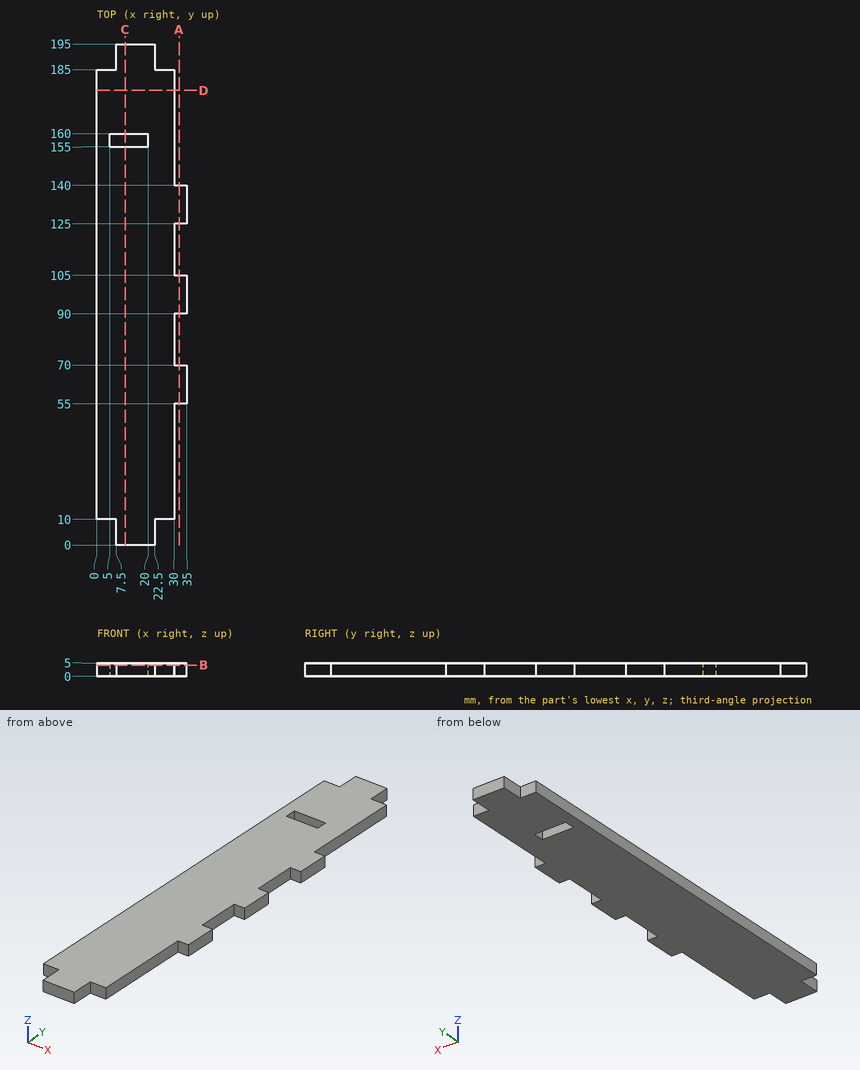
The figure shows three views and two pictorial views of one solid part (mm, origin at its lowest corner). Answer the questions. Give positions to 0.01 mm unless a question says otherwise; leave off trailing zeros. Loops run counter-clockwise (first coordinate to the right, second up) from the corner with the lowest first, then second, coordinate; pieces in that order, holes last. Notation, with made-up numbers: (-3, -3) -> (54, -3) arc R21 ccw to (54, 31) -> close; hole circle Ø9 at (73.25, 68). An arc over 180 degrees is marked (long way). Put each result on its own line as item: value. Start each with the question number.
Item 1: The part is cut by section C-C (x = 11). Give the vertices of the cut face in (y, z), then the cut area to 3 significant figures.
Item 2: The part is cut by section D-D (y = 177). Give the vertices of the cut face in (x, z), then the cut area to 3 significant figures.
Item 3: The part is cut by section B-B (z = 4.25). Give the vertices of the cut face in (x, y), then the cut area to 3 significant figures.
Item 4: Find the intervals of material crossed by L1, parallel to Y at x = 33.5, z = 4.3; L2, parallel to Y at x = 13.5, z = 1.8; L3, parallel to Y at x = 6, z = 1.6, in increasing order. Write a range as [from, to].
Item 5: Each of these flat-tipped pins is pushed along its axis until it touches: P1, Ø2.5, axis at x = 32, z = 3, coming from the -Y side; P2, Ø2, axis at y = 121, z = 4, coming from the +X side; P3, Ø1.5, axis at x = 28, z = 3, coming from the +Y side. Where does it stop, or does it pass through?
Item 6: The part is cut by section A-A (x = 32). Give the vertices of the cut face in (y, z).
Answers below:
1. outline: (0, 0) -> (155, 0) -> (155, 5) -> (0, 5) -> close; (160, 0) -> (195, 0) -> (195, 5) -> (160, 5) -> close
1. area: 950 mm2
2. outline: (0, 0) -> (30, 0) -> (30, 5) -> (0, 5) -> close
2. area: 150 mm2
3. outline: (0, 10) -> (7.5, 10) -> (7.5, 0) -> (22.5, 0) -> (22.5, 10) -> (30, 10) -> (30, 55) -> (35, 55) -> (35, 70) -> (30, 70) -> (30, 90) -> (35, 90) -> (35, 105) -> (30, 105) -> (30, 125) -> (35, 125) -> (35, 140) -> (30, 140) -> (30, 185) -> (22.5, 185) -> (22.5, 195) -> (7.5, 195) -> (7.5, 185) -> (0, 185) -> close; hole (5, 155) -> (20, 155) -> (20, 160) -> (5, 160) -> close
3. area: 5,700 mm2
4. L1: [55, 70], [90, 105], [125, 140]
4. L2: [0, 155], [160, 195]
4. L3: [10, 155], [160, 185]
5. P1: y = 55
5. P2: x = 30
5. P3: y = 185
6. outline: (55, 0) -> (70, 0) -> (70, 5) -> (55, 5) -> close; (90, 0) -> (105, 0) -> (105, 5) -> (90, 5) -> close; (125, 0) -> (140, 0) -> (140, 5) -> (125, 5) -> close
